```python
from build123d import *

# Parameters (mm, degrees)
F2_R     = 5
F3_DEPTH = 13.6
F4_W     = 2
F4_H     = 7.5


with BuildPart() as f1:
    # F0 (on Right) → F1 (revolve)
    with BuildSketch(Plane.YZ):
        Polygon((-40, 4), (-40, 0), (42.4, 0), (42.4, 5), (40.4, 5), (40.4, 8.25), (38.5, 8.25), (38.5, 17.25), (31, 30), (0, 30), (0, 4), align=None)
    revolve(axis=Axis((0, 1.2, 0), (0, 1, 0)))

    # F2 (on face) → F3 (join)
    with BuildSketch(Plane.XZ):
        Circle(F2_R)
    extrude(amount=F3_DEPTH)

    # F4 (on Right) → F5 (revolve)
    with BuildSketch(Plane.YZ):
        with Locations((-14.6, 3.75)):
            Rectangle(F4_W, F4_H)
    revolve(axis=Axis((0, -14.6, 0), (0, 1, 0)))


solid = f1.part
```
Work out the finished part from the listing and answer in its coordinate system (mm). A direction names the side the tool comes from. Round coordinates to 2 decimals unless told otherwise and drop trailing zeros. Loops run counter-clockwise (first coordinate to the right, second up) from the corner with the lowest first, then second, coordinate; pieces in that order, holes last.
(1) The part is cut by section C-C, the plane y = 37. Give the vertices of the cut face in (x, z), and give its area (3 significant figures).
Computed values:
outline: circle Ø39.6 at (0, 0)
area: 1,230 mm2
(2) Each of these flat-tipped pins is pushed along its axis until it touches: P1, Ø12, axis at y = -24.5, z = 12, coming from the +X side; P2, Ø6, axis at y = -11, z = 0.5, coming from the +X side; P3, Ø2, axis at y = 11.5, z = -16, coming from the +X side; P4, Ø5, axis at x = -6.5, y = 16, coming from the -Z side. Where does it stop, or does it pass through?
Computed values:
P1: passes through
P2: stops at x = 7.5
P3: stops at x = 25.98
P4: stops at z = -29.73
(3) The part is cut by section D-D, the plane y = -24.5. Give the vertices of the cut face in (x, z).
Computed values:
outline: circle Ø8 at (0, 0)
(4) Find the intervals of material crossed by L1, parallel to Y at x = -4, z = -5; L2, parallel to Y at x = -1, z = 10.5; L3, parallel to Z at x = 25, y = 9, in increasing order.
Computed values:
L1: y = -15.6 to -13.6, 0 to 40.4
L2: y = 0 to 38.5
L3: z = -16.58 to 16.58
(5) The mould has two halves that part along Y. Classify faces 1 (the flat face through (-5, -13.6, -2)), 2 (the conical face through (-17.62, 38.03, -3.91)), 3 (the cylindrical face through (-3.16, 39.44, 7.62)): pulls with the +Y half, pulls with the -Y half, needs draft (parallel to the pull), parting line crosses it, or undercut.
Computed values:
face 1: undercut
face 2: pulls with the +Y half
face 3: needs draft
(6) The part is cut by section B-B, the plane x = 0. Give the vertices of the cut face in (y, z).
Computed values:
outline: (-40, -4) - (-15.6, -4) - (-15.6, -7.5) - (-13.6, -7.5) - (-13.6, -5) - (0, -5) - (0, -30) - (31, -30) - (38.5, -17.25) - (38.5, -8.25) - (40.4, -8.25) - (40.4, -5) - (42.4, -5) - (42.4, 5) - (40.4, 5) - (40.4, 8.25) - (38.5, 8.25) - (38.5, 17.25) - (31, 30) - (0, 30) - (0, 5) - (-13.6, 5) - (-13.6, 7.5) - (-15.6, 7.5) - (-15.6, 4) - (-40, 4) - close
(7) The part is cut by section A-A, the plane z = 0. Give the vertices of the cut face in (x, y).
Computed values:
outline: (-30, 0) - (-5, 0) - (-5, -13.6) - (-7.5, -13.6) - (-7.5, -15.6) - (-4, -15.6) - (-4, -40) - (4, -40) - (4, -15.6) - (7.5, -15.6) - (7.5, -13.6) - (5, -13.6) - (5, 0) - (30, 0) - (30, 31) - (17.25, 38.5) - (8.25, 38.5) - (8.25, 40.4) - (5, 40.4) - (5, 42.4) - (-5, 42.4) - (-5, 40.4) - (-8.25, 40.4) - (-8.25, 38.5) - (-17.25, 38.5) - (-30, 31) - close
(8) For faces 4 (the cylindrical face through (1.32, 15.28, -29.97)), 5 (the cylindrical face through (-1.08, -6.7, -4.88)), 6 (the flat face through (0, -40, 0)), 7 (the cylindrical face through (-4.88, 41.39, -1.08)), 8 (the flat face through (-3, -15.6, -3)), determine the directions among +Z, -Z, +X, -X, +Y, -Y from which every point of the face is accessible in a straight line to the end or side of a thin tool.
Computed values:
face 4: +Y, -Y
face 5: none
face 6: +Z, -Z, +X, -X, -Y
face 7: +Y
face 8: -Y
